Could you check a few things on this drawing? It's one solid part, dimensions in mm from its lowest x, y, z. A direction names the side the tool comes from. Give positions to 0.01 mm unless a question says otherwise; leave off trailing zeros. Loops run counter-clockwise (first coordinate to the right, second up) from the corner with the lowest first, then second, coordinate; pieces in that order, holes last. Notation, with made-up numbers: M 37,81.5 L 41,81.5 A37 ccw 41,120.5 Z; hole C 33.5,59.5 d3. An arc over 180 degrees is marked long. Answer in a Markdown table with one row per item. Add a question column.
1. I need wall thicknesses on line 1 along X through (y, z) = (11, 2.3); line 2 along Y through (x, z) = (10, 0.4); line 3 along X through (y, z) = (12.75, 2.1) (1 decimal). Which ranges of each line are inside material? Lowest first, please. Write a range as from..to.
2. Which directions (+Z, -Z, +X, -X, +Y, -Y) give clear straight access to the entire face, cutting with the end or side of a thin tool? Please do the marked faces 4 and 5.
3. If we section it at C-C on z = 2.6: Count the separate pieces of the cut face and the enclosed holes in it, then the cut area to 3 significant figures.
4. If we section it at A-A on x = 9: List the corners of the cut face in (y, z) for me (1 decimal).
5. If we section it at B-B on y = 12.5: List the corners of the cut face in (x, z) for me (1 decimal).
6. I'm going to push a flat-ended pin straight in: pin 1 Ø1 at (y, z) = (18.5, 1.5) entering from +X. Where does the tip first touch, or does it pass through?
7. If we section it at D-D on x = 46: List the corners of the cut face in (y, z) for me (1 decimal).
8. Thinking about a two-plate mould opening in Y: for the marked faces 1, 2 and 3, which applies, released by +Y, released by -Y, zero draft, split by the parting line, or undercut?
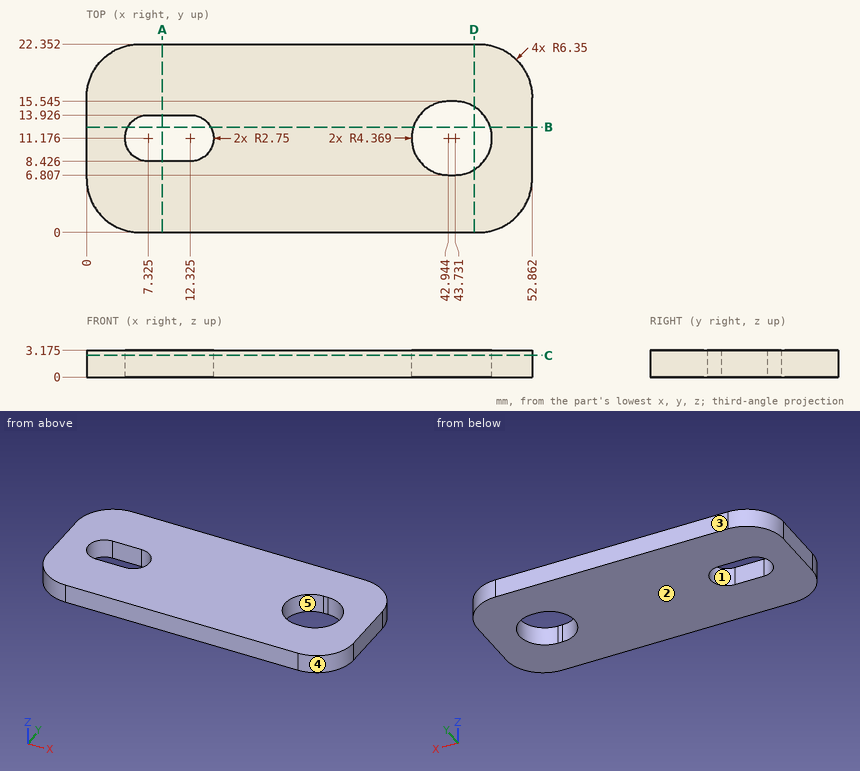
Results:
| question | item | result |
|---|---|---|
| 1 | line 1 | 0..4.58, 15.07..38.58, 48.1..52.86 |
| 1 | line 2 | 0..8.43, 13.93..22.35 |
| 1 | line 3 | 0..5.1, 14.6..38.9, 47.8..52.9 |
| 2 | face 4 | +Z, -Z, +X, -Y |
| 2 | face 5 | +Z, -Z |
| 3 | separate pieces | 1 |
| 3 | enclosed holes | 2 |
| 3 | area | 1,030 mm2 |
| 4 | outline | M 0,0 L 8.4,0 L 8.4,3.2 L 0,3.2 Z; M 13.9,0 L 22.4,0 L 22.4,3.2 L 13.9,3.2 Z |
| 5 | outline | M 0,0 L 4.9,0 L 4.9,3.2 L 0,3.2 Z; M 14.7,0 L 38.8,0 L 38.8,3.2 L 14.7,3.2 Z; M 47.9,0 L 52.9,0 L 52.9,3.2 L 47.9,3.2 Z |
| 6 | pin 1 | x = 52.54 |
| 7 | outline | M 0,0 L 7.4,0 L 7.4,3.2 L 0,3.2 Z; M 14.9,0 L 22.4,0 L 22.4,3.2 L 14.9,3.2 Z |
| 8 | face 1 | undercut |
| 8 | face 2 | zero draft |
| 8 | face 3 | released by +Y |
